```python
from build123d import *

# Parameters (mm, degrees)
BOSS_EXTRUDE1_DEPTH = 44.45
CUT_EXTRUDE1_DEPTH  = 7.35


with BuildPart() as part:
    # Sketch3 → Boss-Extrude1 (new body, symmetric)
    with BuildSketch(Plane(origin=(0, 0, 0), x_dir=(0, 0, -1), z_dir=(1, 0, 0))):
        Polygon((-88.825470595, 3.175), (-85.159296386, -3.175), (60.083377372, -3.175), (71.0819, 3.175), align=None)
    extrude(amount=BOSS_EXTRUDE1_DEPTH, both=True)

    # Sketch5 → Cut-Extrude1 (cut, through all)
    with BuildSketch(Plane(origin=(0, 3.175, 0), x_dir=(1, 0, 0), z_dir=(0, 1, 0))):
        with BuildLine():
            ThreePointArc((-35.56, 71.0819), (0, 35.5219), (35.56, 71.0819))
            Line((35.56, 71.0819), (-35.56, 71.0819))
        make_face()
    extrude(amount=-CUT_EXTRUDE1_DEPTH, mode=Mode.SUBTRACT)


solid = part.part
```
Check sheet for the modelled part. Datum: model origin and axes. Units: mm. Coordinates: 2 decimals unless noted, no trailing zeros. Order: outer loops, then holes, each group sorted by start corner. A loop starts at its lowest first (then second) coordinate and runs counter-clockwise, first axis right, second up. Notation, with made-up numbers: (26, -30.75) -> (55, -30.75) arc R25 cw to (55, -5.75) -> close; hole circle Ø10 at (52, -20). An arc over 180 degrees is marked (long way). Write item = value, one per line. Start each with the question number.
1) Cross-section at C-C (x = -32). Enter the section's corners in (y, z) (3 decimals), then the cut area to 3 significant figures.
2) Cross-section at A-A (y = 0.75). Enter the section's corners in (x, z), then the cut area to 3 significant figures.
3) Mould release check, pull along X, two halves, no side actions. Record for faces 1 (the flat face through (-44.45, 0, 10)), 2 (the flat face through (44.45, 0, 10)), 3 (the flat face through (39.21, -0.04, -65.51)), 4 (the cylindrical face through (-0.78, 0.04, -35.53)): +X half, -X half, draft (parallel to the pull), parting line (faces both ways), or undercut.
4) Material ranges on L1, parallel to X at y = -1.75, z = -41; L2, parallel to X at y = -0.5, z = -48; L3, parallel to Z at x = 27, y = 2, recorded low to high.
5) Cross-section at B-B (x = 0). Enter the section's corners in (y, z) (3 decimals).
6) Go/stop test with a flat-tipped pin: P1, Ø1, axis at x = 23, y = -0.5, coming from the -Z side. Record where the tip stops, or that it passes through.
Ans:
q1.outline = (-3.175, -55.573) -> (3.175, -55.573) -> (3.175, 88.825) -> (-3.175, 85.159) -> close
q1.area = 905 mm²
q2.outline = (-44.45, -66.88) -> (-35.31, -66.88) arc R35.56 cw to (35.31, -66.88) -> (44.45, -66.88) -> (44.45, 87.43) -> (-44.45, 87.43) -> close
q2.area = 12,000 mm²
q3.face_1 = -X half
q3.face_2 = +X half
q3.face_3 = draft
q3.face_4 = undercut
q4.L1 = -44.45 to -18.96, 18.96 to 44.45
q4.L2 = -44.45 to -27.05, 27.05 to 44.45
q4.L3 = -47.94 to 88.15
q5.outline = (-3.175, -35.522) -> (3.175, -35.522) -> (3.175, 88.825) -> (-3.175, 85.159) -> close
q6.P1 = -44.39
